The listing builds one solid part. Answer for the finished solid, in the listing's coordinates (mm). A direction names the side the tool comes from. Round coordinates to 2 decimals unless told otherwise and drop trailing zeros. Order: outer loops, then holes, each group sorted by start corner. A loop starts at its lowest first (then second) coordinate and runs counter-clockwise, first axis right, second up. Notation, with made-up numbers: (59, -27.5) - (87, -27.5) arc R30 ccw to (87, 8.5) - close; hole circle Ø9 at (-21, 1.25). An arc over 180 degrees is marked (long way). Use CSV: the item, a comma, the result in double quotes. Start each with the question number.
Item 1: Find section A-A, the plane y = 0. Give the vertices of the cut face in (x, z).
Item 2: Find section C-C, the plane x = -15. Give the vertices of the cut face in (y, z).
Item 3: For faces 5 (the cylindrical face through (-61.555, -0.133, 5.43)), 6 (the cylindrical face through (-0.484, -2.403, 14.905)), 7 (the cylindrical face through (73.99, 4.71, 6.23)), determine the directions among +Z, -Z, +X, -X, +Y, -Y from which every point of the face is accessible in a straight line to the end or side of a thin tool.
Item 4: Flat-ended cylindrical pins translate along their axes: P1, Ø4, axis at y = 5.5, z = 14, coming from the +X side; P2, Ø8, axis at x = 28, z = 14, coming from the -Y side; P3, Ø1.5, axis at x = -57.5, z = 6, coming from the -Y side; P4, Ø1.5, axis at x = 49, y = 2.5, coming from the -Z side. Find the tip coordinate at first contact, or state that the pin passes through.
Item 5: Determine the mould class of faces 1 (the flat face through (82.03, 0, 7)), 2 (the flat face through (50.254, -6, 10)), 3 (the cylindrical face through (61.15, -0.28, 0.93)), 4 (the cylindrical face through (78.81, -2.356, 14.754)) for opening direction X: +X half, -X half, draft (parallel to the pull), parting line (faces both ways), or undercut.
Item 6: Find section B-B, the plane z = 10. Give the vertices of the cut face in (x, y), plus the area to 3 significant figures.
Item 7: Straight lines are drawn through the part: line 1 along X through (y, z) = (-3, 14); line 2 along X through (y, z) = (5.5, 7.5); line 3 along X through (y, z) = (6.5, 7.75). For each, find the intervals that lie inside material, in ascending order. Write a range as [from, to].
```python
from build123d import *

# Parameters (mm, degrees)
F2_R     = 4.318
F3_DEPTH = 127


with BuildPart() as f1:
    # F0 (on Front) → F1 (revolve)
    with BuildSketch(Plane.XZ):
        Polygon((-75.958224, 16.798637), (-75.958224, 7.273637), (82.029776, 7.273637), (82.029776, 15.115878), (75.679776, 15.115878), (75.679776, 12.099637), (72.352376, 12.099637), (72.352376, 13.623637), (50.254376, 13.623637), (50.254376, 15.274637), (-49.821624, 15.274637), (-49.821624, 13.623637), (-55.384224, 13.623637), (-55.384224, 16.798637), align=None)
    revolve(axis=Axis((3.035776, 0, 7.273637), (1, 0, 0)))

    # F2 (on Front) → F3 (cut, symmetric)
    with BuildSketch(Plane.XZ):
        with Locations((-65.544224, 7.084235)):
            Circle(F2_R)
    extrude(amount=F3_DEPTH, both=True, mode=Mode.SUBTRACT)


solid = f1.part
```
Worked out:
1,outline,"(-75.96, -2.25) - (-55.38, -2.25) - (-55.38, 0.92) - (-49.82, 0.92) - (-49.82, -0.73) - (50.25, -0.73) - (50.25, 0.92) - (72.35, 0.92) - (72.35, 2.45) - (75.68, 2.45) - (75.68, -0.57) - (82.03, -0.57) - (82.03, 15.12) - (75.68, 15.12) - (75.68, 12.1) - (72.35, 12.1) - (72.35, 13.62) - (50.25, 13.62) - (50.25, 15.27) - (-49.82, 15.27) - (-49.82, 13.62) - (-55.38, 13.62) - (-55.38, 16.8) - (-75.96, 16.8) - close; hole circle Ø8.64 at (-65.54, 7.08)"
2,outline,"circle Ø16 at (0, 7.27)"
3,face 5,"+Y, -Y"
3,face 6,"+X"
3,face 7,"none"
4,P1,"stops at x = 82.03"
4,P2,"stops at y = -7.52"
4,P3,"stops at y = -9.51"
4,P4,"stops at z = -0.53"
5,face 1,"+X half"
5,face 2,"undercut"
5,face 3,"undercut"
5,face 4,"draft"
6,outline,"(-75.96, -9.13) - (-68.73, -9.13) - (-68.73, 9.13) - (-75.96, 9.13) - close; (-62.36, -9.13) - (-55.38, -9.13) - (-55.38, -5.73) - (-49.82, -5.73) - (-49.82, -7.52) - (50.25, -7.52) - (50.25, -5.73) - (72.35, -5.73) - (72.35, -3.98) - (75.68, -3.98) - (75.68, -7.35) - (82.03, -7.35) - (82.03, 7.35) - (75.68, 7.35) - (75.68, 3.98) - (72.35, 3.98) - (72.35, 5.73) - (50.25, 5.73) - (50.25, 7.52) - (-49.82, 7.52) - (-49.82, 5.73) - (-55.38, 5.73) - (-55.38, 9.13) - (-62.36, 9.13) - close"
6,area,"2,200 mm²"
7,line 1,"x = [-75.96, -55.38], [-49.82, 50.25], [75.68, 82.03]"
7,line 2,"x = [-75.96, -69.84], [-61.25, 72.35], [75.68, 82.03]"
7,line 3,"x = [-75.96, -69.81], [-61.28, -55.38], [-49.82, 50.25], [75.68, 82.03]"
